Verification items for the finished model (mm, model axes). A direction names the side the tool comes from. Coordinates: 2 decimals unless noted, no trailing zeros. Order: outer loops, then holes, each group sorted by start corner. A loop starts at its lowest first (then second) coordinate and runs counter-clockwise, first axis right, second up. Notation, with made-up numbers: M 57,41.25 L 115,41.25 A21 ccw 115,47.25 Z; hole C 15,38 d8. An arc over 180 degrees is marked long. Return JSON: item names as keys, results as strings. Group by question number.
1. Mould release check, pull along X, two halves, no side actions. Record for faces 3 (the flat face through (-0.8, -6, 15)), 4 (the flat face through (0, -12.75, 12)): +X half, -X half, draft (parallel to the pull), parting line (faces both ways), or undercut.
2. Section check B-B, the plane y = 6.75. Record the cut outline in (x, z).
3. Section check C-C, the plane x = 8.5. Record the cut outline in (y, z).
4. Section check A-A, the plane z = 22.25. Record the cut outline in (x, y).
5. Set-up check for faces 1 (the flat face through (0, 0, 0)), 2 (the flat face through (-17.25, -6, 15)): record each of +Z, -Z, +X, -X, +Y, -Y from which the full face is reachable in a straight line by a thin tool's end or side.
6. Material ranges on line 1 along Y through (x, z) = (-1, 19); line 2 along X through (y, z) = (1, 5.25); line 3 along Z through (x, y) = (-7, -1), recorded low to high.
7. Gauge pin test, flat end, axial feed: pin 1 (3 mm diameter, centred on x = -12.5, y = 7, fed in from +Z). Record the tip position at first contact, or that the pin passes through.
```python
from build123d import *

# Parameters (mm, degrees)
F0_W     = 38
F0_H     = 25.5
F1_DEPTH = 25
F2_W     = 34.5
F2_H     = 22
F3_DEPTH = 20
F4_W     = 16.45
F4_H     = 1.6
F4_W_2   = 1.6
F4_H_2   = 10.2
F5_DEPTH = 20


with BuildPart() as f1:
    # F0 (on Top) → F1 (new body)
    with BuildSketch(Plane.XY):
        Rectangle(F0_W, F0_H)
    extrude(amount=F1_DEPTH)

    # F2 (on face) → F3 (cut)
    with BuildSketch(Plane.XY.offset(25)):
        Rectangle(F2_W, F2_H)
    extrude(amount=-F3_DEPTH, mode=Mode.SUBTRACT)

    # F4 (on face) → F5 (join)
    with BuildSketch(Plane.XY.offset(5)):
        with Locations((-9.025, 0)):
            Rectangle(F4_W, F4_H)
        with Locations((0, -5.9)):
            Rectangle(F4_W_2, F4_H_2)
        Rectangle(F4_W_2, F4_H)
        with Locations((0, 5.9)):
            Rectangle(F4_W_2, F4_H_2)
        with Locations((9.025, 0)):
            Rectangle(F4_W, F4_H)
    extrude(amount=F5_DEPTH)


solid = f1.part
```
Answers follow:
{
 "1": {"face 3": "undercut", "face 4": "draft"},
 "2": {"outline": "M -19,0 L 19,0 L 19,25 L 17.25,25 L 17.25,5 L 0.8,5 L 0.8,25 L -0.8,25 L -0.8,5 L -17.25,5 L -17.25,25 L -19,25 Z"},
 "3": {"outline": "M -12.75,0 L 12.75,0 L 12.75,25 L 11,25 L 11,5 L 0.8,5 L 0.8,25 L -0.8,25 L -0.8,5 L -11,5 L -11,25 L -12.75,25 Z"},
 "4": {"outline": "M -19,-12.75 L 19,-12.75 L 19,12.75 L -19,12.75 Z; hole M -17.25,-11 L -0.8,-11 L -0.8,-0.8 L -17.25,-0.8 Z; hole M -17.25,0.8 L -0.8,0.8 L -0.8,11 L -17.25,11 Z; hole M 0.8,-11 L 17.25,-11 L 17.25,-0.8 L 0.8,-0.8 Z; hole M 0.8,0.8 L 17.25,0.8 L 17.25,11 L 0.8,11 Z"},
 "5": {"face 1": "-Z, +X, -X, +Y, -Y", "face 2": "+Z"},
 "6": {"line 1": "-12.75 to -11, -0.8 to 0.8, 11 to 12.75", "line 2": "-19 to -17.25, -0.8 to 0.8, 17.25 to 19", "line 3": "0 to 5"},
 "7": {"pin 1": "z = 5"}
}
